Source: CAD feature listing. Evaluate the final solid. Frame: model axes, mm. Give positions to 0.01 mm unless a question says otherwise; leave off trailing zeros. Order: outer loops, then holes, each group sorted by start corner. A loop starts at its lowest first (then second) coordinate and runs counter-clockwise, first axis right, second up. Notation, with made-up numbers: (0, 69) - (4, 69) arc R18 ccw to (4, 95) - close; hole circle Ø4 at (84.25, 88.5). An arc over 180 degrees is marked (long way). One line per item, written item: value. Start each with the question number.
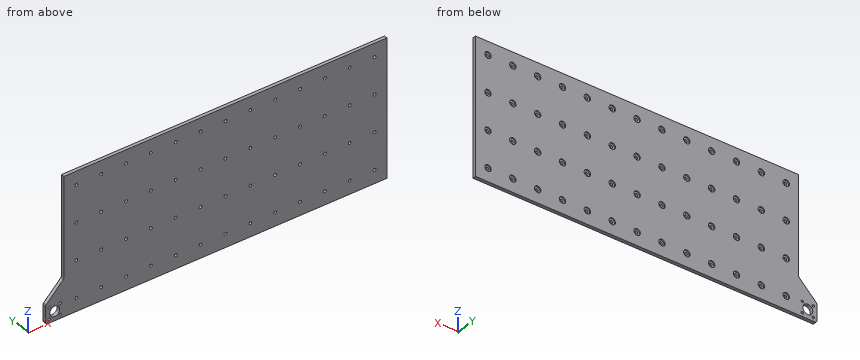
from build123d import *

# Parameters (mm, degrees)
SKETCH1_R            = 2.25
SKETCH1_R_2          = 9.5
BOSS_EXTRUDE1_DEPTH  = 6.35
FILLET1_R            = 4
HOLE1_D              = 5.5
HOLE1_CBORE_D        = 12.24
HOLE1_CBORE_DEPTH    = 2.38125
LPATTERN1_COUNT      = 13
LPATTERN1_PITCH      = 47.4
LPATTERN1_COUNT_DIR2 = 4
LPATTERN1_PITCH_DIR2 = 69


with BuildPart() as part:
    # Sketch1 → Boss-Extrude1 (new body)
    with BuildSketch(Plane(origin=(0, 0, 0), x_dir=(1, 0, 0), z_dir=(0, 1, 0))):
        Polygon((-35, 222.2), (0, 187.2), (0, 0), (616.2, 0), (616.2, 257.2), (0, 257.2), (-35, 257.2), align=None)
        with Locations(Location((-28, 229.2, 0), (0, 0, 270))):
            Circle(SKETCH1_R, mode=Mode.SUBTRACT)
        with Locations(Location((-7, 229.2, 0), (0, 0, 270))):
            Circle(SKETCH1_R, mode=Mode.SUBTRACT)
        with Locations(Location((-7, 250.2, 0), (0, 0, 270))):
            Circle(SKETCH1_R, mode=Mode.SUBTRACT)
        with Locations(Location((-28, 250.2, 0), (0, 0, 270))):
            Circle(SKETCH1_R, mode=Mode.SUBTRACT)
        with Locations(Location((-17.5, 239.7, 0), (0, 0, 270))):
            Circle(SKETCH1_R_2, mode=Mode.SUBTRACT)
    extrude(amount=BOSS_EXTRUDE1_DEPTH)

    # Fillet1
    fillet1_edges = [part.edges().sort_by_distance(p)[0] for p in [
        (0, 3.175, -187.2),
        (-35, 3.175, -222.2),
        (-35, 3.175, -257.2),
    ]]
    fillet(fillet1_edges, radius=FILLET1_R)

    # Hole1 (through all)
    with Locations(Plane(origin=(0, 6.35, 0), x_dir=(1, 0, 0), z_dir=(0, 1, 0))):
        with Locations((23.7, 25.1)):
            hole1 = CounterBoreHole(HOLE1_D / 2, HOLE1_CBORE_D / 2, HOLE1_CBORE_DEPTH)

    # LPattern1: Hole1 13 × 4
    with Locations(*[(i * LPATTERN1_PITCH, 0, -j * LPATTERN1_PITCH_DIR2) for i in range(LPATTERN1_COUNT) for j in range(LPATTERN1_COUNT_DIR2) if (i, j) != (0, 0)]):
        add(hole1, mode=Mode.SUBTRACT)


solid = part.part
1. Section A-A on y = 1. Count the separate pieces of the cut face and the enclosed holes in it, then the cut area to 3 significant figures.
2. Ray query, L1, parallel to Z at x = 118.5, y = 5.7; L2, parallel to Z at x = 165.9, y = 1.25; L3, parallel to X at y = 2, z = -229.2. Return the intervals inside material, ascending.
3. Section B-B on z = -49.5. Return the cut outline in (x, y), then the cut area to 3 significant figures.
4. Contact query for flat-ended pins moving along their axis: pin 1 Ø3.5 at (x, z) = (119.5, -92.5) entering from +Y; pin 2 Ø1 at (y, z) = (3, -167) entering from -X. Output: stop coordinate, or through.
Data:
1. separate pieces: 1
1. enclosed holes: 57
1. area: 159,000 mm2
2. L1: z = -257.2 to -238.22, -225.98 to -169.22, -156.98 to -100.22, -87.98 to -31.22, -18.98 to 0
2. L2: z = -257.2 to -234.85, -229.35 to -165.85, -160.35 to -96.85, -91.35 to -27.85, -22.35 to 0
2. L3: x = -35 to -30.25, -25.75 to -9.25, -4.75 to 616.2
3. outline: (0, 0) - (616.2, 0) - (616.2, 6.35) - (0, 6.35) - close
3. area: 3,910 mm2
4. pin 1: stops at y = 3.97
4. pin 2: stops at x = 0
